```python
from build123d import *

# Parameters (mm, degrees)
F0_R     = 50.8
F0_R_2   = 37.8
F1_DEPTH = 2
F2_DEPTH = 13
F3_R     = 12.99999


# Not quite as in the source:
# - a fillet or chamfer is up to 0.001 mm smaller than in the source, because OpenCascade refuses the exact size


with BuildPart() as f1:
    # F0 (on Top) → F1 (new body)
    with BuildSketch(Plane.XY):
        Circle(F0_R)
        Circle(F0_R_2, mode=Mode.SUBTRACT)
        Circle(F0_R_2)
    extrude(amount=-F1_DEPTH)

    # F0 (on Top) → F2 (join)
    with BuildSketch(Plane.XY):
        Circle(F0_R)
        Circle(F0_R_2, mode=Mode.SUBTRACT)
    extrude(amount=F2_DEPTH)

    # F3 (radius 13 in the source; OpenCascade refuses exactly that, so slightly less here)
    f3_edges = [f1.edges().sort_by_distance(p)[0] for p in [
        (-50.8, 0, 13),
    ]]
    fillet(f3_edges, radius=F3_R)


solid = f1.part
```
Could you check a few things on this model? Use its own coordinates, in mm. Coordinates: 2 decimals unless noted, no trailing zeros. Order: outer loops, then holes, each group sorted by start corner. A loop starts at its lowest first (then second) coordinate and runs counter-clockwise, first axis right, second up. Notation, with made-up numbers: M 75.25,-34 L 88.25,-34 A30 cw 88.25,-5 Z; hole C -40,17.5 d8. An arc over 180 degrees is marked long. Use a Markdown table: item, result. Add a question column.
Q1. I'm going to push flat-ended pins straight in: pin 1 (3 mm diameter, centred on y = -19, z = 9, fed in from -X); pin 2 (8 mm diameter, centred on x = -17, z = 9.5, fed in from +Y); pin 3 (1 mm diameter, centred on x = -20, z = 6.5, fed in from +Y). Where does each tip first touch, or does it pass through?
Q2. I want a section at C-C on z = 9. List the corners of the cut face in (x, y) for me, then the cut area to 3 significant figures.
Q3. I want a section at D-D on z = 3.75. List the corners of the cut face in (x, y) for me, then the cut area to 3 significant figures.
Q4. If I drill on L1, parallel to Z at x = -28, y = 5.5; L2, parallel to Y at x = 0, z = 4.25; L3, parallel to X at y = 17.5, z = 5, over which ranges is the centre line in solid material (lowest first)?
Q5. We'd pull the mould along X, two halves only. Please class faces 1 (the flat face through (-1, 1, 0)), 2 (the flat face through (-1, 1, -2)): pulls with the +X half, pulls with the -X half, needs draft (parallel to the pull), parting line crosses it, or undercut.
Checked values:
| question | item | result |
|---|---|---|
| 1 | pin 1 | x = -44.69 |
| 1 | pin 2 | y = 46.98 |
| 1 | pin 3 | y = 45.17 |
| 2 | outline | C 0,0 d94.36; hole C 0,0 d75.6 |
| 2 | area | 2,500 mm² |
| 3 | outline | C 0,0 d100.49; hole C 0,0 d75.6 |
| 3 | area | 3,440 mm² |
| 4 | L1 | -2 to 0 |
| 4 | L2 | -50.09 to -37.8, 37.8 to 50.09 |
| 4 | L3 | -46.62 to -33.51, 33.51 to 46.62 |
| 5 | face 1 | undercut |
| 5 | face 2 | needs draft |
